Could you check a few things on this model? Use its own coordinates, in mm. Face numbers are marked on the shaded views. A direction names the side the tool comes from. Round coordinates to 2 decimals unless told otherwise and drop trailing zeros. Loops run counter-clockwise (first coordinate to the right, second up) from the corner with the lowest first, then second, coordinate; pieces in that order, holes last. Notation, with made-up numbers: (58.5, -21.5) -> (111.5, -21.5) arc R23 ccw to (111.5, -8.5) -> close; hole circle Ø9 at (36, 21). An arc over 180 degrees is marked (long way). One line per item, written item: value.
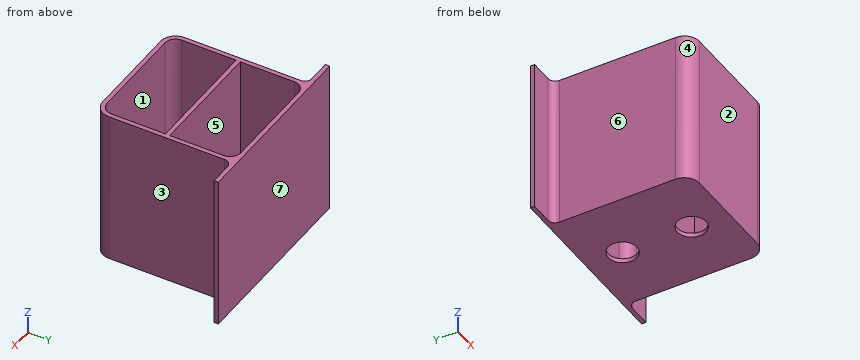
```python
from build123d import *

# Parameters (mm, degrees)
F0_W          = 33
F0_H          = 1.2
F1_DEPTH      = 42
F1_DEPTH_BACK = 1.2
F0_R          = 4
F2_DEPTH      = 1.2
F3_R          = 2


with BuildPart() as f1:
    # F0 (on Top) → F1 (new body, two sides)
    with BuildSketch(Plane.XY) as f1_sk:
        with BuildLine():
            Line((-17.7, 15.6), (-17.7, -15.6))
            ThreePointArc((-17.7, -15.6), (-16.469848, -18.569848), (-13.5, -19.8))
            Line((-13.5, -19.8), (13.5, -19.8))
            ThreePointArc((13.5, -19.8), (16.469848, -18.569848), (17.7, -15.6))
            Line((17.7, -15.6), (17.7, 15.6))
            Line((17.7, 15.6), (17.7, 18.6))
            Line((17.7, 18.6), (26, 18.6))
            Line((26, 18.6), (26, 19.8))
            Line((26, 19.8), (-26, 19.8))
            Line((-26, 19.8), (-26, 18.6))
            Line((-26, 18.6), (-17.7, 18.6))
            Line((-17.7, 18.6), (-17.7, 15.6))
        make_face()
        with BuildLine():
            ThreePointArc((16.5, -15.6), (15.62132, -17.72132), (13.5, -18.6))
            Line((13.5, -18.6), (-13.5, -18.6))
            ThreePointArc((-13.5, -18.6), (-15.62132, -17.72132), (-16.5, -15.6))
            Line((-16.5, -15.6), (-16.5, -0.6))
            Line((-16.5, -0.6), (-16.5, 0.6))
            Line((-16.5, 0.6), (-16.5, 15.6))
            ThreePointArc((-16.5, 15.6), (-15.62132, 17.72132), (-13.5, 18.6))
            Line((-13.5, 18.6), (13.5, 18.6))
            ThreePointArc((13.5, 18.6), (15.62132, 17.72132), (16.5, 15.6))
            Line((16.5, 15.6), (16.5, 0.6))
            Line((16.5, 0.6), (16.5, -0.6))
            Line((16.5, -0.6), (16.5, -15.6))
        make_face(mode=Mode.SUBTRACT)
        Rectangle(F0_W, F0_H)
    extrude(amount=F1_DEPTH)
    extrude(f1_sk.sketch, amount=-F1_DEPTH_BACK)

    # F0 (on Top) → F2 (join)
    with BuildSketch(Plane.XY):
        with BuildLine():
            Line((-16.5, 0.6), (16.5, 0.6))
            Line((16.5, 0.6), (16.5, 15.6))
            ThreePointArc((16.5, 15.6), (15.62132, 17.72132), (13.5, 18.6))
            Line((13.5, 18.6), (-13.5, 18.6))
            ThreePointArc((-13.5, 18.6), (-15.62132, 17.72132), (-16.5, 15.6))
            Line((-16.5, 15.6), (-16.5, 0.6))
        make_face()
        with Locations((0, 9.6)):
            Circle(F0_R, mode=Mode.SUBTRACT)
        Rectangle(F0_W, F0_H)
        with BuildLine():
            Line((-13.5, -18.6), (13.5, -18.6))
            ThreePointArc((13.5, -18.6), (15.62132, -17.72132), (16.5, -15.6))
            Line((16.5, -15.6), (16.5, -0.6))
            Line((16.5, -0.6), (-16.5, -0.6))
            Line((-16.5, -0.6), (-16.5, -15.6))
            ThreePointArc((-16.5, -15.6), (-15.62132, -17.72132), (-13.5, -18.6))
        make_face()
        with Locations((0, -9.6)):
            Circle(F0_R, mode=Mode.SUBTRACT)
    extrude(amount=-F2_DEPTH)

    # F3
    f3_edges = [f1.edges().sort_by_distance(p)[0] for p in [
        (-17.7, 18.6, 20.4),
        (17.7, 18.6, 20.4),
    ]]
    fillet(f3_edges, radius=F3_R)


solid = f1.part
```
(1) On a 3-axis mill with a long thin cutter (end or side, diameter ignored), from which of +Z, -Z, +X, -X, +Y, -Y can I reach the whole of each face in a straight line? I mean the marked faces 5, 6 and 7. Say none if no direction works.
Results below:
face 5: +Z
face 6: +Z, -Z, -X, -Y
face 7: +Z, -Z, +X, -X, +Y
(2) For pin 1 Ø12 at (y, z) = (-5.5, 21.5) entering from -X; pin 2 Ø2 at (y, z) = (10, 31.5) entering from +X; pin 3 Ø7 at (x, y) = (0, 9.6) entering from -Z (3 decimals); pin 4 Ø10 at (x, y) = (-5, -7) entering from +Z, each with a flat end and sliding along its axis, tell me the tip position at first contact or that it passes through.
Results below:
pin 1: stops at x = -17.7
pin 2: stops at x = 17.7
pin 3: passes through
pin 4: stops at z = 0
(3) Imagine slicing it at D-D on y = -14.5. Write out the boundary of the cut face in (x, z), then the cut area to 3 significant figures.
Results below:
outline: (-17.7, -1.2) -> (17.7, -1.2) -> (17.7, 42) -> (16.5, 42) -> (16.5, 0) -> (-16.5, 0) -> (-16.5, 42) -> (-17.7, 42) -> close
area: 143 mm²
(4) Imagine slicing it at C-C on z = 20. Write out the boundary of the cut face in (x, y).
Results below:
outline: (-26, 18.6) -> (-19.7, 18.6) arc R2 cw to (-17.7, 16.6) -> (-17.7, -15.6) arc R4.2 ccw to (-13.5, -19.8) -> (13.5, -19.8) arc R4.2 ccw to (17.7, -15.6) -> (17.7, 16.6) arc R2 cw to (19.7, 18.6) -> (26, 18.6) -> (26, 19.8) -> (-26, 19.8) -> close; hole (-16.5, -15.6) arc R3 ccw to (-13.5, -18.6) -> (13.5, -18.6) arc R3 ccw to (16.5, -15.6) -> (16.5, -0.6) -> (-16.5, -0.6) -> close; hole (-16.5, 0.6) -> (16.5, 0.6) -> (16.5, 15.6) arc R3 ccw to (13.5, 18.6) -> (-13.5, 18.6) arc R3 ccw to (-16.5, 15.6) -> close
(5) Please list where these lines run through material, in increasing order: L1, parallel to Y at x = -7, z = 20.5; L2, parallel to Y at x = 0, z = -0.3; L3, parallel to X at y = -15, z = 7.
Results below:
L1: y = -19.8 to -18.6, -0.6 to 0.6, 18.6 to 19.8
L2: y = -19.8 to -13.6, -5.6 to 5.6, 13.6 to 19.8
L3: x = -17.7 to -16.5, 16.5 to 17.7
(6) Imagine slicing it at A-A on y = 9.6. Write out the boundary of the cut face in (x, z), then the cut area to 3 significant figures.
Results below:
outline: (-17.7, -1.2) -> (-4, -1.2) -> (-4, 0) -> (-16.5, 0) -> (-16.5, 42) -> (-17.7, 42) -> close; (4, -1.2) -> (17.7, -1.2) -> (17.7, 42) -> (16.5, 42) -> (16.5, 0) -> (4, 0) -> close
area: 134 mm²
(7) Imagine slicing it at B-B on x = 0. Write out the boundary of the cut face in (y, z), then the cut area to 3 significant figures.
Results below:
outline: (-19.8, -1.2) -> (-13.6, -1.2) -> (-13.6, 0) -> (-18.6, 0) -> (-18.6, 42) -> (-19.8, 42) -> close; (-5.6, -1.2) -> (5.6, -1.2) -> (5.6, 0) -> (0.6, 0) -> (0.6, 42) -> (-0.6, 42) -> (-0.6, 0) -> (-5.6, 0) -> close; (13.6, -1.2) -> (19.8, -1.2) -> (19.8, 42) -> (18.6, 42) -> (18.6, 0) -> (13.6, 0) -> close
area: 180 mm²
(8) We'd pull the mould along X, two halves only. Please class the marked faces 1, 2, 3 and 4: +X half, -X half, draft (parallel to the pull), parting line (faces both ways), or undercut.
Results below:
face 1: undercut
face 2: draft
face 3: +X half
face 4: -X half
